Could you check a few things on this drawing? It's one solid part, dimensions in mm from its lowest x, y, z. A direction names the side the tool comes from. Round coordinates to 2 decimals unless told otherwise and drop trailing zeros. Write each loop counter-clockwise with the first axis right and the second up, starting at its lowest first coordinate (ties: lowest second). Pieces come first, ordered by that corner, then holes. Notation, with made-up numbers: M 87.5,85.5 L 111.5,85.5 A27 cw 111.5,121.5 Z; hole C -35,11.25 d3. An arc over 180 degrees is marked long. One line per item, written item: value. Start each with the question number.
(1) Thinking about a two-plate mould opening in Z: for the marked faces 3, 4 and 5, which applies, released by +Z, released by -Z, zero draft, split by the parting line, or undercut?
(2) I want a section at B-B on z = 22. Please give me the cut outline in (x, y) (3 decimals), and give its area (3 significant figures).
(3) I'm going to push a flat-ended pin straight in: pin 1 Ø3.5 at (x, z) = (79.5, 11.5) entering from +Y. Where does the tip first touch, or does it pass through?
(4) I want a section at A-A on x = 115. Please give me the cut outline in (y, z).
(5) Which directions (+Z, -Z, +X, -X, +Y, -Y) give clear straight access to the entire face, cutting with the end or side of a thin tool? Please do the marked faces 1 and 2.
(6) If I drill on L1, parallel to Y at x = 44.5, z = 5; L2, parallel to Y at x = 15.5, z = 19, over which ranges is the centre line in solid material (lowest first)?
(7) I want a section at C-C on x = 27. Please give me the cut outline in (y, z), and give its area (3 significant figures).
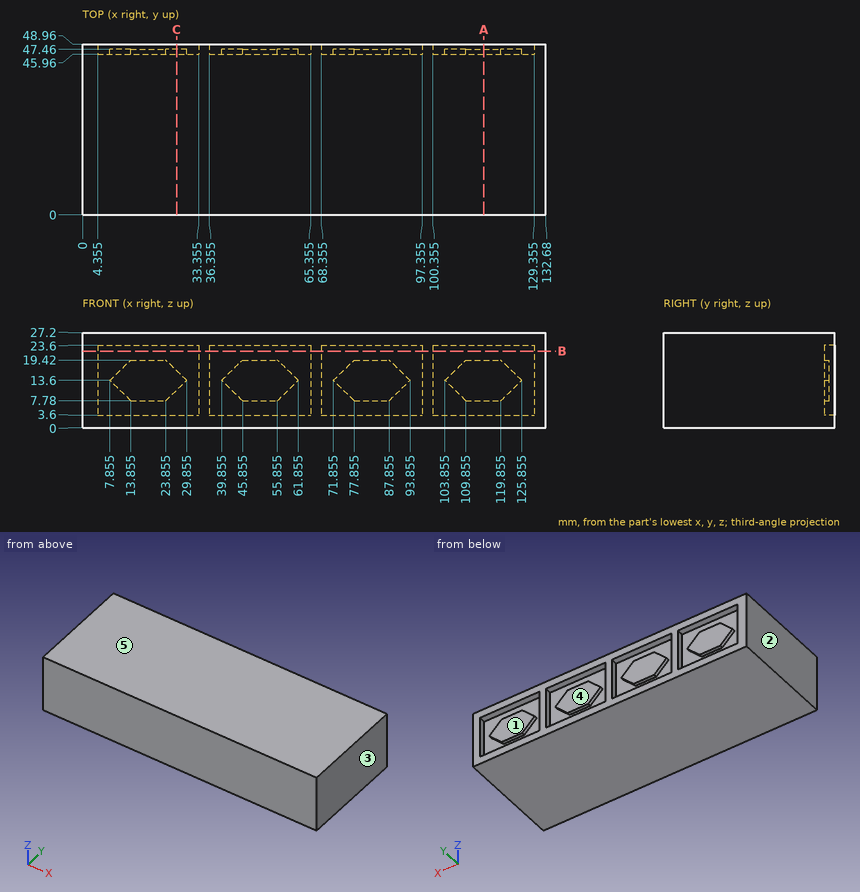
Found:
1. face 3: zero draft
1. face 4: undercut
1. face 5: released by +Z
2. outline: M 0,0 L 132.68,0 L 132.68,48.96 L 129.355,48.96 L 129.355,45.96 L 100.355,45.96 L 100.355,48.96 L 97.355,48.96 L 97.355,45.96 L 68.355,45.96 L 68.355,48.96 L 65.355,48.96 L 65.355,45.96 L 36.355,45.96 L 36.355,48.96 L 33.355,48.96 L 33.355,45.96 L 4.355,45.96 L 4.355,48.96 L 0,48.96 Z
2. area: 6,150 mm²
3. pin 1: stops at y = 47.46
4. outline: M 0,0 L 48.96,0 L 48.96,3.6 L 45.96,3.6 L 45.96,7.78 L 47.46,7.78 L 47.46,19.42 L 45.96,19.42 L 45.96,23.6 L 48.96,23.6 L 48.96,27.2 L 0,27.2 Z
5. face 1: +Y
5. face 2: +Z, -Z, -X, +Y, -Y
6. L1: y = 0 to 45.96
6. L2: y = 0 to 47.46
7. outline: M 0,0 L 48.96,0 L 48.96,3.6 L 45.96,3.6 L 45.96,10.83 L 47.46,10.83 L 47.46,16.37 L 45.96,16.37 L 45.96,23.6 L 48.96,23.6 L 48.96,27.2 L 0,27.2 Z
7. area: 1,280 mm²
